from build123d import *

# Parameters (mm, degrees)
SALIENTE_EXTRUIR1_DEPTH = 35
CROQUIS9_W              = 60
CROQUIS9_H              = 10
SALIENTE_EXTRUIR2_DEPTH = 0.975


with BuildPart() as part:
    # Croquis1 → Saliente-Extruir1 (new body)
    with BuildSketch(Plane.XY):
        Polygon((-1.95, -0.7), (-1.95, 0.7), (-0.975, 0.7), (-0.975, 1.9), (0.975, 1.9), (0.975, 0.7), (1.95, 0.7), (1.95, -0.7), align=None)
    extrude(amount=-SALIENTE_EXTRUIR1_DEPTH)

    # Croquis9 → Saliente-Extruir2 (add, symmetric)
    with BuildSketch(Plane(origin=(0, 0, 0), x_dir=(0, 0, -1), z_dir=(1, 0, 0))):
        with Locations((30, 6.9)):
            Rectangle(CROQUIS9_W, CROQUIS9_H)
    extrude(amount=SALIENTE_EXTRUIR2_DEPTH, both=True)


solid = part.part
Part model, mm, in its own coordinate system. A direction names the side the tool comes from. Round coordinates to 2 decimals unless told otherwise and drop trailing zeros. Loops run counter-clockwise (first coordinate to the right, second up) from the corner with the lowest first, then second, coordinate; pieces in that order, holes last. Notation, with made-up numbers: (-12.75, 52.25) - (-2.75, 52.25) arc R9 cw to (-2.75, 56.25) - close; hole circle Ø4 at (82, -1). An arc over 180 degrees is marked (long way). Answer as a JSON object with one key per item and string values.
Item 1: Tool access for faces 1 (the face through (0.975, 6, -30)), 2 (the face through (-0.975, 6, -30)), 3 (the face through (0, 1.9, -47)): list every direction of +Z, -Z, +X, -X, +Y, -Y with a clear straight run to the whole face (end or side of a thin tool).
Output:
{"face 1": "+Z, -Z, +X, +Y", "face 2": "+Z, -Z, -X, +Y", "face 3": "-Z, +X, -X, -Y"}
Item 2: Band-saw the part on C-C on y = 3. List the corners of the cut face in (x, z) (3 decimals).
Output:
{"outline": "(-0.975, -60) - (0.975, -60) - (0.975, 0) - (-0.975, 0) - close"}
Item 3: Band-saw the part on A-A on z = -13. List the corners of the cut face in (x, y) (3 decimals).
Output:
{"outline": "(-1.95, -0.7) - (1.95, -0.7) - (1.95, 0.7) - (0.975, 0.7) - (0.975, 11.9) - (-0.975, 11.9) - (-0.975, 0.7) - (-1.95, 0.7) - close"}
Item 4: Band-saw the part on B-B on x = -0.05. List the corners of the cut face in (y, z), plus the area to 3 significant figures.
Output:
{"outline": "(-0.7, -35) - (1.9, -35) - (1.9, -60) - (11.9, -60) - (11.9, 0) - (-0.7, 0) - close", "area": "691 mm2"}
Item 5: Band-saw the part on D-D on z = -42.5. List the corners of the cut face in (x, y) (3 decimals), plus the area to 3 significant figures.
Output:
{"outline": "(-0.975, 1.9) - (0.975, 1.9) - (0.975, 11.9) - (-0.975, 11.9) - close", "area": "19.5 mm2"}
Item 6: Wall check: L1, parallel to X at y = 5, z = -55 (3 decimals); L2, parallel to Y at x = -1.7, z = -32.5; L3, parallel to Z at x = -0.9, y = 0.75. Give the ranges that are in metal, low to high.
Output:
{"L1": "-0.975 to 0.975", "L2": "-0.7 to 0.7", "L3": "-35 to 0"}
Item 7: Pin check, flat tips, straight feed: pin 1 (2 mm diameter, centred on y = 9.5, z = -52, fed in from +X) (3 decimals); pin 2 (1.5 mm diameter, centred on y = 1.5, z = -9.5, fed in from -X) (3 decimals); pin 3 (2 mm diameter, centred on x = 0, y = 0.5, fed in from -Z). Stop position of each tip, or through.
Output:
{"pin 1": "x = 0.975", "pin 2": "x = -0.975", "pin 3": "z = -35"}
